Can you work these out from the model? Positions are in its coordinate system, mm. Face numbers are marked on the shaded views. A direction names the side the tool comes from. Coordinates: 2 decimals unless noted, no trailing zeros. Order: outer loops, then holes, each group sorted by start corner. A loop starts at its lowest first (then second) coordinate and runs counter-clockwise, first axis right, second up. Notation, with made-up numbers: (55, 70.5) -> (69, 70.5) arc R18 cw to (69, 95.5) -> close; hole circle Ø2 at (23, 11). An arc over 180 degrees is marked (long way). Answer as a JSON object with one key per item and string values. Group by question number.
(1) I want a section at A-A, the plane y = 0.5. List the corners of the cut face in (x, z) for me.
(2) I need wall thicknesses on line 1 (Y direction, x = -0.4, z = 0.15); line 2 (Y direction, x = 0.5, z = -1.15); line 3 (Z direction, x = 0.5, y = 7.75). Which ranges of each line are inside material? Lowest first, please.
(3) Which directions (+Z, -Z, +X, -X, +Y, -Y) give clear straight access to the entire face, cutting with the end or side of a thin tool? Please do the marked faces 1 and 2.
(4) For pin 1 (0.5 mm diameter, centred on x = 0, y = -1.5, fed in from +Z); pin 2 (1.5 mm diameter, centred on x = 1, y = 5.5, fed in from -Z), each with a flat end and sliding along its axis, tell me the tip position at first contact or that it passes through.
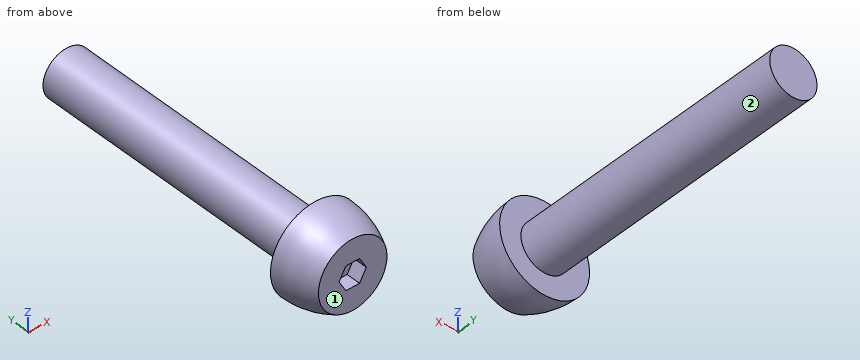
from build123d import *

# Parameters (mm, degrees)
SKETCH_1_R          = 1
EXTRUDE_375_DEPTH   = 12
EXTRUDE_START       = -1.8
SKETCH_1_3_R        = 1.9
SKETCH_1_3_R_2      = 1
EXTRUDE_453_DEPTH   = 1.8
CUT_EXTRUDE_1_DEPTH = 0.6


with BuildPart() as part:
    # 草图1 → Extrude 375 (new body)
    with BuildSketch(Plane(origin=(0, 0, 0), x_dir=(1, 0, 0), z_dir=(0, 1, 0))):
        with Locations(Location((0, 0, 0), (0, 0, 270))):
            Circle(SKETCH_1_R)
    extrude(amount=EXTRUDE_375_DEPTH)

    # 草图1<3> → Extrude 453 (add)
    # profile 1 of 2: a face of its own
    with BuildSketch(Plane(origin=(0, 0, 0), x_dir=(1, 0, 0), z_dir=(0, 1, 0)).offset(EXTRUDE_START)):
        with Locations(Location((0, 0, 0), (0, 0, 270))):
            Circle(SKETCH_1_3_R)
        with Locations(Location((0, 0, 0), (0, 0, 270))):
            Circle(SKETCH_1_3_R_2, mode=Mode.SUBTRACT)
    # profile 2 of 2: a face of its own
    with BuildSketch(Plane(origin=(0, 0, 0), x_dir=(1, 0, 0), z_dir=(0, 1, 0)).offset(EXTRUDE_START)):
        with Locations(Location((0, 0, 0), (0, 0, 270))):
            Circle(SKETCH_1_3_R_2)
    extrude(amount=EXTRUDE_453_DEPTH)

    # 草图2 → 切除-旋转1 (revolve, cut)
    with BuildSketch(Plane.XY, mode=Mode.PRIVATE) as cut_revolve_1_sk:
        with BuildLine():
            Line((-1.9, 0), (-1.9, -1.8))
            Line((-1.9, -1.8), (-1.45, -1.8))
            ThreePointArc((-1.45, -1.8), (-1.785795063, -0.927698766), (-1.9, 0))
        make_face()
    revolve(cut_revolve_1_sk.sketch.rotate(Axis((0, 0, 0), (0, 1, 0)), 90), axis=Axis((0, 0, 0), (0, 1, 0)), mode=Mode.SUBTRACT)

    # 草图3 → 切除-拉伸1 (cut)
    with BuildSketch(Plane.XZ.offset(1.8)):
        Polygon((-0.288675135, -0.5), (0.288675135, -0.5), (0.577350269, 0), (0.288675135, 0.5), (-0.288675135, 0.5), (-0.577350269, 0), align=None)
    extrude(amount=-CUT_EXTRUDE_1_DEPTH, mode=Mode.SUBTRACT)


solid = part.part
Computed values:
{
 "1": {"outline": "circle Ø2 at (0, 0)"},
 "2": {"line 1": "y = -1.2 to 12", "line 2": "y = -1.8 to 0", "line 3": "z = -0.87 to 0.87"},
 "3": {"face 1": "+Z, -Z, +X, -X, -Y", "face 2": "+Y"},
 "4": {"pin 1": "stops at z = 1.69", "pin 2": "stops at z = -0.97"}
}
